Input: dimensioned drawing with shaded views. Units: mm. Origin: part minimum x, y, z. A direction names the side the tool comes from. Coordinates: 2 decimals unless noted, no trailing zeros. Loops run counter-clockwise (first coordinate to the right, second up) from the corner with the lowest first, then second, coordinate; pieces in that order, holes last.
Item 1: Section C-C on y = 5. Return loops of the section in (x, z).
Item 2: Section B-B on z = 43.5. Return loops of the section in (x, y), and give its area (3 significant figures).
Item 3: Section A-A on x = 94.5. Return loops of the section in (y, z), and give its area (3 significant figures).
Item 4: Reachability of the marked faces 1, 2 and 3 from +Z, -Z, +X, -X, +Y, -Y: full face, straight path, thin tool, end or side. Return the list, or none.
Item 5: Contact query for flat-ended pins moving along their axis: P1, Ø4, axis at x = 34, y = 30.5, coming from the -Z side; P2, Ø5, axis at x = 35, z = 31.5, coming from the +Y side; P3, Ø4, axis at x = 48.5, z = 7, coming from the +Y side; P4, Ø5, axis at x = 14, z = 46, coming from the -Y side. Output: stop coordinate, or through.
Item 6: Pull-direction query (Y, two-part tool) for the marked faces 4, 5, 6 and 7; classes: released by +Y, released by -Y, zero draft, split by the parting line, or undercut.
Item 7: Section D-D on y = 48. Return loops of the section in (x, z).
Item 8: Ray query, line 1 along Y through (x, z) = (6, 36.5); line 2 along Y through (x, z) = (31.5, 46); line 3 along Z through (x, y) = (62, 24). Return the intervals inside material, ascending.
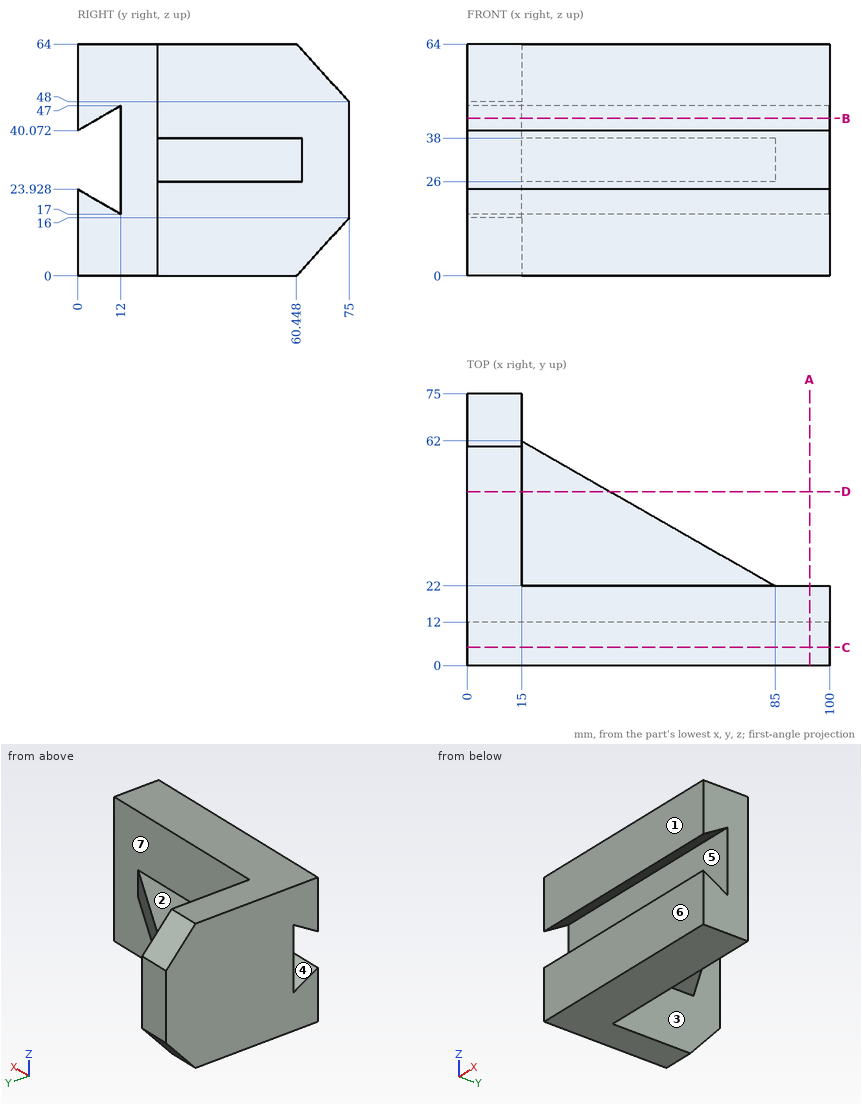
Results found:
1. outline: (0, 0) - (100, 0) - (100, 21.04) - (0, 21.04) - close; (0, 42.96) - (100, 42.96) - (100, 64) - (0, 64) - close
2. outline: (0, 0) - (100, 0) - (100, 5.94) - (0, 5.94) - close; (0, 12) - (100, 12) - (100, 22) - (15, 22) - (15, 75) - (0, 75) - close
2. area: 2,390 mm2
3. outline: (0, 0) - (22, 0) - (22, 64) - (0, 64) - (0, 40.07) - (12, 47) - (12, 17) - (0, 23.93) - close
3. area: 1,130 mm2
4. face 1: +Z, -Z, +X, -X, -Y
4. face 2: +Z, +X, +Y
4. face 3: +X, +Y
5. P1: stops at z = 26
5. P2: stops at y = 52
5. P3: stops at y = 22
5. P4: stops at y = 0
6. face 4: undercut
6. face 5: undercut
6. face 6: released by -Y
6. face 7: released by +Y
7. outline: (0, 0) - (15, 0) - (15, 26) - (39.5, 26) - (39.5, 38) - (15, 38) - (15, 64) - (0, 64) - close
8. line 1: y = 12 to 75
8. line 2: y = 0 to 10.27, 12 to 22
8. line 3: z = 26 to 38
